Source: CAD feature listing. Evaluate the final solid. Frame: model axes, mm. Coordinates: 2 decimals unless noted, no trailing zeros. Order: outer loops, then holes, each group sorted by start corner. A loop starts at its lowest first (then second) coordinate and runs counter-clockwise, first axis right, second up.
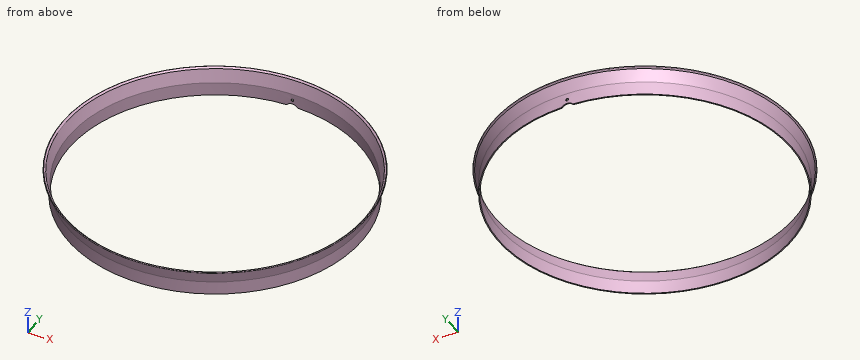
```python
from build123d import *

# Parameters (mm, degrees)
SKETCH8_R          = 1.5
CUT_EXTRUDE1_DEPTH = 675.332492822


with BuildPart() as part:
    # Sketch1 → Revolve1 (revolve)
    with BuildSketch(Plane(origin=(-300, 0, 0), x_dir=(0, -1, 0), z_dir=(-1, 0, 0)), mode=Mode.PRIVATE) as revolve1_sk:
        with BuildLine():
            Line((-631.585161389, -424.526276491), (-635.785161389, -438.713521565))
            Line((-635.785161389, -438.713521565), (-635.785161389, -453.670006409))
            Line((-635.785161389, -453.670006409), (-634.585161389, -453.670006409))
            Line((-634.585161389, -453.670006409), (-634.585161389, -438.785397411))
            Line((-634.585161389, -438.785397411), (-630.582706756, -425.265443891))
            ThreePointArc((-630.582706756, -425.265443891), (-629.96855649, -424.639289663), (-629.250787995, -424.135247944))
            ThreePointArc((-629.250787995, -424.135247944), (-629.005156259, -423.410467755), (-629.571265705, -422.895529538))
            ThreePointArc((-629.571265705, -422.895529538), (-630.666584798, -423.601768681), (-631.585161389, -424.526276491))
        make_face()
    revolve(revolve1_sk.sketch.rotate(Axis((-300, 798.285161389, -417.264314325), (0, 0, -1)), 90), axis=Axis((-300, 798.285161389, -417.264314325), (0, 0, -1)))

    # Sketch8 → Cut-Extrude1 (cut, through all)
    with BuildSketch(Plane(origin=(0, 798.285161389, 0), x_dir=(1, 0, 0), z_dir=(0, 1, 0))):
        with Locations(Location((-300, 446.236353344, 0), (0, 0, 90))):
            Circle(SKETCH8_R)
        with BuildLine():
            Line((-293.808705408, 453.670006409), (-306.191294592, 453.670006409))
            ThreePointArc((-306.191294592, 453.670006409), (-300, 450.736353344), (-293.808705408, 453.670006409))
        make_face()
    extrude(amount=CUT_EXTRUDE1_DEPTH, mode=Mode.SUBTRACT)


solid = part.part
```
1. Section query A-A, the plane z = -431.5. Output: boundary loops of the cut face in (x, y), plus the area to 3 significant figures.
2. Contact query for flat-ended pins moving along their axis: P1, Ø8, axis at x = -407.5, z = -439, coming from the +Y side; P2, Ø3, axis at x = -348.5, z = -446.5, coming from the -Y side; P3, Ø1.5, axis at x = -362, z = -437, coming from the -Y side. Output: stop coordinate, or through.
3. Material intervals for line 1 along Y through (x, z) = (-300, -449.75); line 2 along X through (y, z) = (771, -437.5); line 3 along X through (y, z) = (704.5, -427.5), sorted ascending.
Answer key:
1. outline: circle Ø331.71 at (-300, 798.29); hole circle Ø329.27 at (-300, 798.29)
1. area: 1,270 mm2
2. P1: stops at y = 925.37
2. P2: stops at y = 641.48
2. P3: stops at y = 645.82
3. line 1: y = 634.59 to 635.79, 960.79 to 961.99
3. line 2: x = -461.8 to -460.56, -139.44 to -138.2
3. line 3: x = -438.23 to -436.75, -163.25 to -161.77
